Geometry check sheet. Reference: the model listing, model coordinates, mm. Face numbers are marked on the shaded views. A direction names the side the tool comes from. Coordinates: 2 decimals unless noted, no trailing zeros. Loops run counter-clockwise (first coordinate to the right, second up) from the corner with the lowest first, then second, coordinate; pieces in that order, holes last.
from build123d import *

# Parameters (mm, degrees)
SKETCH_W        = 1.9
SKETCH_H        = 5
PAD_DEPTH       = 90
SKETCH001_W     = 2
SKETCH001_H     = 69
SKETCH001_H_2   = 73
POCKET_DEPTH    = 5
SKETCH002_W     = 60.2
SKETCH002_H     = 11.5
PAD001_DEPTH    = 2
SKETCH004_W     = 2
SKETCH004_H     = 2
PAD002_DEPTH    = 4
PAD003_DEPTH    = 92
SKETCH006_W     = 2
SKETCH006_H     = 73
PAD004_DEPTH    = 5
SKETCH007_W     = 2
SKETCH007_H     = 92
PAD005_DEPTH    = 38.74
SKETCH008_W     = 15
SKETCH008_H     = 73
POCKET001_DEPTH = 2
SKETCH009_W     = 2
SKETCH009_H     = 23
PAD006_DEPTH    = 38.74
SKETCH010_W     = 56.2
SKETCH010_H     = 2
PAD007_DEPTH    = 42.74
SKETCH011_W     = 56.2
SKETCH011_H     = 22
POCKET002_DEPTH = 2
SKETCH012_W     = 2
SKETCH012_H     = 15
PAD008_DEPTH    = 69
SKETCH013_W     = 2
SKETCH013_H     = 15
PAD009_DEPTH    = 90
PAD010_DEPTH    = 65


with BuildPart() as part:
    # Sketch → Pad (new body)
    with BuildSketch(Plane.XZ):
        Polygon((-30.1, 0), (30.1, 0), (30.1, 15.5), (28.1, 15.5), (28.1, 2), (-28.1, 2), (-28.1, 15.5), (-30.1, 15.5), align=None)
        with Locations((0, 4.5)):
            Rectangle(SKETCH_W, SKETCH_H)
        with Locations((-20.05, 4.5)):
            Rectangle(SKETCH_W, SKETCH_H)
        with Locations((20.05, 4.5)):
            Rectangle(SKETCH_W, SKETCH_H)
    extrude(amount=PAD_DEPTH)

    # Sketch001 (on Face3 of Pad) → Pocket (cut)
    with BuildSketch(Plane(origin=(0, 0, 15.5), x_dir=(-1, 0, 0), z_dir=(0, 0, 1))):
        with Locations((29.1, 55.5)):
            Rectangle(SKETCH001_W, SKETCH001_H)
        with Locations((-29.1, 53.5)):
            Rectangle(SKETCH001_W, SKETCH001_H_2)
    extrude(amount=-POCKET_DEPTH, mode=Mode.SUBTRACT)

    # Sketch002 (on Face2 of Pocket) → Pad001 (join)
    with BuildSketch(Plane(origin=(0, 0, 0), x_dir=(1, 0, 0), z_dir=(0, 1, 0))):
        with Locations((0, -5.75)):
            Rectangle(SKETCH002_W, SKETCH002_H)
    extrude(amount=PAD001_DEPTH)

    # Sketch004 → Pad002 (join)
    with BuildSketch(Plane(origin=(0, 0, 11.5), x_dir=(-1, 0, 0), z_dir=(0, 0, 1))):
        with Locations((-29.1, -1)):
            Rectangle(SKETCH004_W, SKETCH004_H)
        with Locations((29.1, -1)):
            Rectangle(SKETCH004_W, SKETCH004_H)
    extrude(amount=PAD002_DEPTH)

    # Sketch005 (on Face26 of Pad002) → Pad003 (join)
    with BuildSketch(Plane(origin=(0, 2, 0), x_dir=(1, 0, 0), z_dir=(0, 1, 0))):
        Polygon((-30.1, -54.24), (-30.1, 0), (-32.1, 0), (-32.1, -14.24), (-34.6, -14.24), (-34.6, -12.31), (-36.03, -12.31), (-37.995757, -14.275757), (-37.995757, -19.965757), (-36.03, -21.931514), (-34.6, -21.931514), (-34.6, -20), (-32.1, -20), (-32.1, -34.24), (-34.6, -34.24), (-34.6, -32.31), (-36.03, -32.31), (-37.995757, -34.275757), (-37.995757, -39.965757), (-36.03, -41.931514), (-34.6, -41.931514), (-34.6, -40.001514), (-32.1, -40.001514), (-32.1, -54.24), align=None)
    extrude(amount=-PAD003_DEPTH)

    # Sketch006 (on Face46 of Pad003) → Pad004 (join)
    with BuildSketch(Plane(origin=(0, 0, 10.5), x_dir=(-1, 0, 0), z_dir=(0, 0, 1))):
        with Locations((-29.1, 53.5)):
            Rectangle(SKETCH006_W, SKETCH006_H)
    extrude(amount=PAD004_DEPTH)

    # Sketch007 (on Face48 of Pad004) → Pad005 (join)
    with BuildSketch(Plane(origin=(0, 0, 15.5), x_dir=(-1, 0, 0), z_dir=(0, 0, 1))):
        with Locations((-29.1, 44)):
            Rectangle(SKETCH007_W, SKETCH007_H)
    extrude(amount=PAD005_DEPTH)

    # Sketch008 (on Face48 of Pad005) → Pocket001 (cut)
    with BuildSketch(Plane(origin=(30.1, 0, 0), x_dir=(0, 0, 1), z_dir=(1, 0, 0))):
        with Locations((18, 51.5)):
            Rectangle(SKETCH008_W, SKETCH008_H)
    extrude(amount=-POCKET001_DEPTH, mode=Mode.SUBTRACT)

    # Sketch009 (on Face51 of Pocket001) → Pad006 (join)
    with BuildSketch(Plane(origin=(0, 0, 15.5), x_dir=(-1, 0, 0), z_dir=(0, 0, 1))):
        with Locations((29.1, 9.5)):
            Rectangle(SKETCH009_W, SKETCH009_H)
    extrude(amount=PAD006_DEPTH)

    # Sketch010 (on Face17 of Pad006) → Pad007 (join)
    with BuildSketch(Plane(origin=(0, 0, 11.5), x_dir=(-1, 0, 0), z_dir=(0, 0, 1))):
        with Locations((0, -1)):
            Rectangle(SKETCH010_W, SKETCH010_H)
    extrude(amount=PAD007_DEPTH)

    # Sketch011 (on Face47 of Pad007) → Pocket002 (cut)
    with BuildSketch(Plane.XZ):
        with Locations((0, 22.5)):
            Rectangle(SKETCH011_W, SKETCH011_H)
    extrude(amount=-POCKET002_DEPTH, mode=Mode.SUBTRACT)

    # Sketch012 (on Face49 of Pocket002) → Pad008 (join)
    with BuildSketch(Plane.XZ.offset(21)):
        with Locations((-29.1, 46.74)):
            Rectangle(SKETCH012_W, SKETCH012_H)
    extrude(amount=PAD008_DEPTH)

    # Sketch013 (on Face22 of Pad008) → Pad009 (join)
    with BuildSketch(Plane.XZ):
        with Locations((27.1, 46.74)):
            Rectangle(SKETCH013_W, SKETCH013_H)
    extrude(amount=PAD009_DEPTH)

    # Sketch014 (on Face44 of Pad009) → Pad010 (join)
    with BuildSketch(Plane.XZ):
        Polygon((20.32, 39.24), (20.32, 43.44), (22.12, 43.44), (22.12, 41.24), (23.92, 41.24), (26.118204, 43.44), (26.118204, 39.24), align=None)
        Polygon((20.32, 54.24), (20.32, 50.04), (22.12, 50.04), (22.12, 52.24), (23.92, 52.24), (26.118204, 50.04), (26.118204, 54.24), align=None)
        Polygon((-22.32, 43.44), (-22.32, 39.24), (-28.12, 39.24), (-28.12, 43.438204), (-25.92, 41.24), (-24.12, 41.24), (-24.12, 43.44), align=None)
        Polygon((-22.32, 54.24), (-22.32, 50.04), (-24.12, 50.04), (-24.12, 52.24), (-25.92, 52.24), (-28.118204, 50.04), (-28.118204, 54.24), align=None)
    extrude(amount=PAD010_DEPTH)


solid = part.part
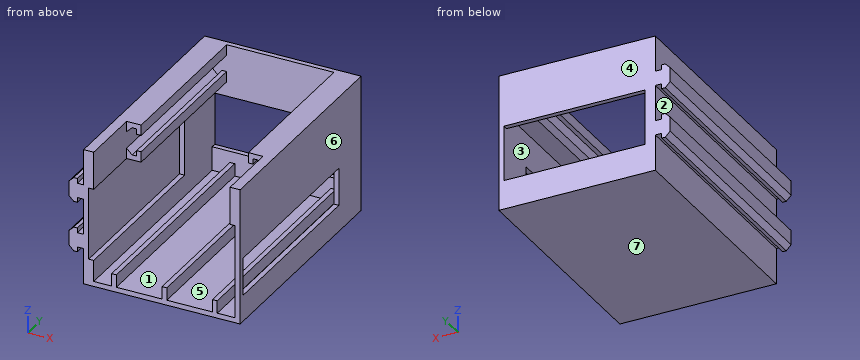
1) Depth check by flat-ended pin: pin 1 (1.6 mm diameter, centred on x = -35.5, y = -30, fed in from +Z); pin 2 (8 mm diameter, centred on x = 19.5, y = -73, fed in from -Z); pin 3 (5 mm diameter, centred on x = 21.5, y = -76.5, fed in from +Z); pin 4 (4 mm diameter, centred on y = -27, z = 3.5, fed in from -X). Enter the tip coordinate at first touch or a pass-through.
Data:
pin 1: stops at z = 41.93
pin 2: stops at z = 0
pin 3: stops at z = 7
pin 4: stops at x = -32.1
2) Section check C-C on z = 36. Record the cut outline in (x, y).
Data:
outline: (-38, -90) - (-30.1, -90) - (-30.1, -21) - (-28.1, -21) - (-28.1, 0) - (28.1, 0) - (28.1, -90) - (30.1, -90) - (30.1, 2) - (-38, 2) - close
3) Section check B-B on x = -17.5. Record the cut outline in (y, z).
Data:
outline: (-90, 0) - (2, 0) - (2, 11.5) - (0, 11.5) - (0, 2) - (-90, 2) - close; (0, 33.5) - (2, 33.5) - (2, 54.24) - (0, 54.24) - close
4) Section check A-A on z = 30. Record the cut outline in (x, y), and give its area (3 significant figures).
Data:
outline: (-32.1, -90) - (-30.1, -90) - (-30.1, -21) - (-28.1, -21) - (-28.1, 2) - (-32.1, 2) - close; (28.1, -90) - (30.1, -90) - (30.1, 2) - (28.1, 2) - close
area: 414 mm2
5) Material ranges on probe 1 along X at (y, z) = (-75.5, 6); probe 2 along Z at (x, y) = (-22.5, -42); probe 3 along X at (y, z) = (-35, 38), recorded low to high.
Data:
probe 1: x = -32.1 to -28.1, -21 to -19.1, -0.95 to 0.95, 19.1 to 21, 28.1 to 30.1
probe 2: z = 0 to 2, 39.24 to 43.44, 50.04 to 54.24
probe 3: x = -38 to -30.1, 28.1 to 30.1
6) Access from +Z, -Z, +X, -X, +Y, -Y to the whole of each face (thin tool, end or side, straight path). Record for the marked faces 1, 2, 3 and 4.
Data:
face 1: +Z, -Y
face 2: +Y, -Y
face 3: -Y
face 4: +Z, -Z, +X, -X, +Y
7) Mould release check, pull along X, two halves, no side actions. Record for the marked faces 5, 6 and 7: +X half, -X half, draft (parallel to the pull), parting line (faces both ways), or undercut.
Data:
face 5: undercut
face 6: +X half
face 7: draft
